Build history of the part. All positions in model axes, mm. Round coordinates to 2 decimals unless told otherwise and drop trailing zeros. Write each loop counter-clockwise with the first axis right and the second up, starting at its lowest first coordinate (ties: lowest second). Pieces come first, ordered by that corner, then holes.
from build123d import *

# Parameters (mm, degrees)
BOSS_EXTRU_1_DEPTH      = 4
ESQUISSE2_R             = 1.25
ENL_V_MAT_EXTRU_1_DEPTH = 14.458268834


with BuildPart() as part:
    # Esquisse1 → Boss.-Extru.1 (new, symmetric)
    with BuildSketch(Plane(origin=(0, 0, 0), x_dir=(1, 0, 0), z_dir=(0, 1, 0))):
        with BuildLine():
            Line((-7.335700376, 2.5), (-1.658312395, 2.5))
            ThreePointArc((-1.658312395, 2.5), (0, -3), (1.658312395, 2.5))
            Line((1.658312395, 2.5), (7.335700376, 2.5))
            ThreePointArc((7.335700376, 2.5), (0, -7.75), (-7.335700376, 2.5))
        make_face()
    extrude(amount=BOSS_EXTRU_1_DEPTH, both=True)

    # Esquisse2 → Enlèv. mat.-Extru.1 (cut, through all)
    with BuildSketch(Plane(origin=(0, 0, -2.5), x_dir=(-1, 0, 0), z_dir=(0, 0, -1))):
        with Locations((-5, 0)):
            Circle(ESQUISSE2_R)
        with Locations((5, 0)):
            Circle(ESQUISSE2_R)
    extrude(amount=-ENL_V_MAT_EXTRU_1_DEPTH, mode=Mode.SUBTRACT)


solid = part.part
1) Slice it at C-C (x = 5). Write the cut outline in (y, z), plus the area to 3 significant figures.
Results:
outline: (-4, -2.5) - (-1.25, -2.5) - (-1.25, 5.92) - (-4, 5.92) - close; (1.25, -2.5) - (4, -2.5) - (4, 5.92) - (1.25, 5.92) - close
area: 46.3 mm2
2) Mould opens along Y. For faces 1 (the flat face through (0, 4, 4)), 2 (the cylindrical face through (0, 0, 3)), 3 (the cylindrical face through (3.81, 0.38, 2.08)) say: released by +Y, released by -Y, zero draft, split by the parting line, or undercut.
Results:
face 1: released by +Y
face 2: zero draft
face 3: undercut
3) Wall check: L1, parallel to Z at x = 2.5, y = 3.75; L2, parallel to X at y = 0, z = 1; L3, parallel to X at y = 0, z = 0.5. Give the ranges that are in metal, low to high.
Results:
L1: z = -2.5 to -1.66, 1.66 to 7.34
L2: x = -7.69 to -6.25, -3.75 to -2.83, 2.83 to 3.75, 6.25 to 7.69
L3: x = -7.73 to -6.25, -3.75 to -2.96, 2.96 to 3.75, 6.25 to 7.73
4) Pin check, flat tip, straight feed: pin 1 Ø3 at (x, y) = (-5, 0) entering from -Z. Stop position of the tip, or through.
Results:
pin 1: stops at z = -2.5
5) Slice it at D-D (z = 1.5). Write the cut outline in (x, y).
Results:
outline: (-7.6, -4) - (-2.6, -4) - (-2.6, 4) - (-7.6, 4) - close; (2.6, -4) - (7.6, -4) - (7.6, 4) - (2.6, 4) - close; hole circle Ø2.5 at (-5, 0); hole circle Ø2.5 at (5, 0)
6) Slice it at B-B (y = 0). Write the cut outline in (x, z), plus the area to 3 significant figures.
Results:
outline: (-7.34, -2.5) - (-6.25, -2.5) - (-6.25, 4.58) arc R7.75 ccw to start; (-3.75, -2.5) - (-1.66, -2.5) arc R3 cw (long way) to (1.66, -2.5) - (3.75, -2.5) - (3.75, 6.78) arc R7.75 ccw to (-3.75, 6.78) - close; (6.25, -2.5) - (7.34, -2.5) arc R7.75 ccw to (6.25, 4.58) - close
area: 63.5 mm2
7) Slice it at A-A (z = 0). Write the cut outline in (x, y).
Results:
outline: (-7.75, -4) - (-3, -4) - (-3, 4) - (-7.75, 4) - close; (3, -4) - (7.75, -4) - (7.75, 4) - (3, 4) - close; hole circle Ø2.5 at (-5, 0); hole circle Ø2.5 at (5, 0)
